CAD build for the part. Positions are in the model's coordinates, mm. A direction names the side the tool comes from. Coordinates: 2 decimals unless noted, no trailing zeros. Order: outer loops, then holes, each group sorted by start corner. A loop starts at its lowest first (then second) coordinate and runs counter-clockwise, first axis right, second up. Notation, with made-up numbers: M -4.75,33.5 L 27.25,33.5 A15 ccw 27.25,53.5 Z; hole C -14.75,17 d3. An arc over 180 degrees is marked long. One line per item, written item: value.
from build123d import *

# Parameters (mm, degrees)
SKETCH_1_R          = 26.75
SKETCH_1_R_2        = 21.75
EXTRUDE_1_DEPTH     = 1
SKETCH_2_W          = 5.751238768
SKETCH_2_H          = 20.704459562
CUT_EXTRUDE_1_DEPTH = 10
FILLET_1_R          = 2
SKETCH_3_R          = 1
CUT_EXTRUDE_2_DEPTH = 10


with BuildPart() as part:
    # 草图1 → 拉伸-薄壁1 (new body)
    with BuildSketch(Plane.XY):
        Circle(SKETCH_1_R)
        Circle(SKETCH_1_R_2, mode=Mode.SUBTRACT)
    extrude(amount=EXTRUDE_1_DEPTH)

    # 草图2 → 切除-拉伸1 (cut)
    with BuildSketch(Plane.XY.offset(1)):
        with Locations((0, 17.972621147)):
            Rectangle(SKETCH_2_W, SKETCH_2_H)
    extrude(amount=-CUT_EXTRUDE_1_DEPTH, mode=Mode.SUBTRACT)

    # 圆角1
    fillet_1_edges = [part.edges().sort_by_distance(p)[0] for p in [
        (2.875619384, 21.559065684, 0.5),
        (-2.875619384, 21.559065684, 0.5),
    ]]
    fillet(fillet_1_edges, radius=FILLET_1_R)

    # 草图3 → 切除-拉伸2 (cut)
    with BuildSketch(Plane.XY.offset(1)):
        with Locations((-4.807050905, 23.823279289)):
            Circle(SKETCH_3_R)
        with Locations((4.807050905, 23.823279289)):
            Circle(SKETCH_3_R)
    extrude(amount=-CUT_EXTRUDE_2_DEPTH, mode=Mode.SUBTRACT)


solid = part.part
Q1. Drill centre lines: line 1 along X through (y, z) = (-0.5, 0.5); line 2 along X through (y, z) = (-2.5, 0.75); line 3 along Y through (x, z) = (-13, 0.15). Where is each one in solid material? Low to high.
Recorded:
line 1: x = -26.75 to -21.74, 21.74 to 26.75
line 2: x = -26.63 to -21.61, 21.61 to 26.63
line 3: y = -23.38 to -17.44, 17.44 to 23.38
Q2. Slice it at B-B (x = 11). List the corners of the cut face in (y, z).
Recorded:
outline: M -24.38,0 L -18.76,0 L -18.76,1 L -24.38,1 Z; M 18.76,0 L 24.38,0 L 24.38,1 L 18.76,1 Z
Q3. Pin check, flat tip, straight feed: pin 1 Ø12 at (x, y) = (-12.5, 1.5) entering from +Z. Stop position of the tip, or through.
Recorded:
pin 1: passes through
Q4. Slice it at A-A (y = 0). List the corners of the cut face in (x, z), plus the area to 3 significant figures.
Recorded:
outline: M -26.75,0 L -21.75,0 L -21.75,1 L -26.75,1 Z; M 21.75,0 L 26.75,0 L 26.75,1 L 21.75,1 Z
area: 10.0 mm^2
Q5. Slice it at C-C (z = 0.25). List the corners of the cut face in (x, y), plus the area to 3 significant figures.
Recorded:
outline: M -4.47,21.29 A2 ccw -2.88,23.24 L -2.88,26.59 A26.75 ccw long 2.88,26.59 L 2.88,23.24 A2 ccw 4.47,21.29 A21.75 cw long Z; hole C -4.81,23.82 d2; hole C 4.81,23.82 d2
area: 726 mm^2
Q6. Which spindle directions (+Z, -Z, +X, -X, +Y, -Y) get a long thin tool onto all of the face, cutting with end or side? Do faces 1 (the face through (-3.335, 21.969, 0.493)), 2 (the face through (-4, -22, 0)). Say none if no direction does.
Recorded:
face 1: +Z, -Z
face 2: -Z, +X, -X, +Y, -Y
Q7. Mould opens along Y. For faces 3 (the face through (-1.136, -26.726, 0.493)), 4 (the face through (-4, -22, 1)), 5 (the face through (-4.937, 24.815, 0.507)) say: released by +Y, released by -Y, zero draft, split by the parting line, or undercut.
Recorded:
face 3: split by the parting line
face 4: zero draft
face 5: undercut
Q8. Slice it at D-D (x = 0). List the corners of the cut face in (y, z), plus the area to 3 significant figures.
Recorded:
outline: M -26.75,0 L -21.75,0 L -21.75,1 L -26.75,1 Z
area: 5.00 mm^2
